Print and shaded views of the part. All mm, measured from the part's lowest x, y and z. Round coordinates to 2 decimals unless told otherwise and drop trailing zeros. Write each loop counter-clockwise with the first axis right and the second up, starting at its lowest first coordinate (ties: lowest second). Pieces come first, ordered by that corner, then holes. Notation, with made-up numbers: (-13.5, 61) - (36.5, 61) arc R7 cw to (36.5, 72) - close; hole circle Ø7 at (38.25, 65). An arc over 180 degrees is marked (long way). One line per item, written item: value.
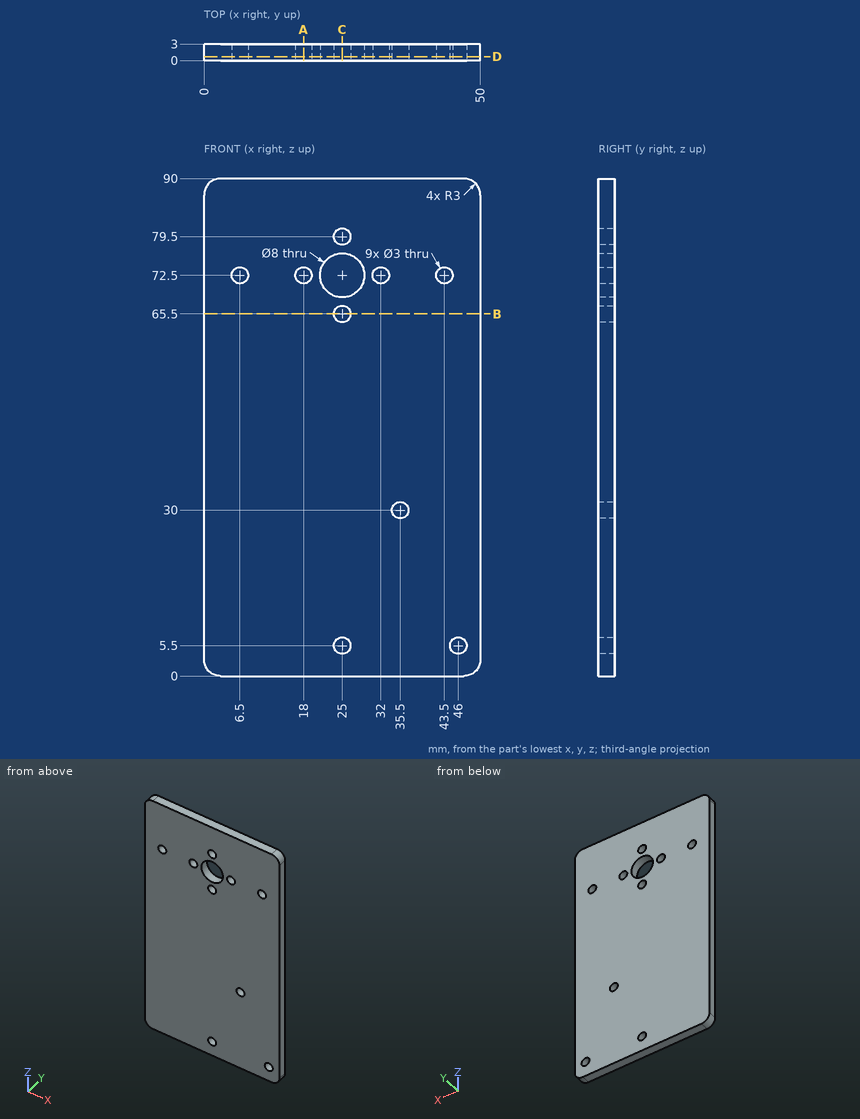
1. Wall check: probe 1 along X at (y, z) = (0.75, 72.5); probe 2 along X at (y, z) = (1.1, 5.5); probe 3 along X at (y, z) = (1.4, 30). Give the ranges that are in metal, low to high. Write a range as [from, to].
Report:
probe 1: [0, 5], [8, 16.5], [19.5, 21], [29, 30.5], [33.5, 42], [45, 50]
probe 2: [0, 23.5], [26.5, 44.5], [47.5, 50]
probe 3: [0, 34], [37, 50]
2. Band-saw the part on C-C on x = 25. Write the cut outline in (y, z).
Report:
outline: (0, 0) - (3, 0) - (3, 4) - (0, 4) - close; (0, 7) - (3, 7) - (3, 64) - (0, 64) - close; (0, 67) - (3, 67) - (3, 68.5) - (0, 68.5) - close; (0, 76.5) - (3, 76.5) - (3, 78) - (0, 78) - close; (0, 81) - (3, 81) - (3, 90) - (0, 90) - close
3. Drop flat-ended pins along their axis: pin 1 (4 mm diameter, centred on x = 25, z = 79.5, fed in from +Y); pin 2 (1.8 mm diameter, centred on x = 25, z = 65.5, fed in from -Y). Give the stop position or say it passes through.
Report:
pin 1: y = 3
pin 2: through
4. Band-saw the part on A-A on x = 18. Write the cut outline in (y, z), plus the area to 3 significant figures.
Report:
outline: (0, 0) - (3, 0) - (3, 71) - (0, 71) - close; (0, 74) - (3, 74) - (3, 90) - (0, 90) - close
area: 261 mm²
5. Band-saw the part on B-B on z = 65.5. Write the cut outline in (x, y).
Report:
outline: (0, 0) - (23.5, 0) - (23.5, 3) - (0, 3) - close; (26.5, 0) - (50, 0) - (50, 3) - (26.5, 3) - close
6. Band-saw the part on D-D on y = 0.7. State how many separate pieces and enclosed holes the cut face has, plus the area to 3 significant figures.
Report:
separate pieces: 1
enclosed holes: 10
area: 4,380 mm²
